Can you work these out from the drawing? Everything is in mm from the part's minimum corner. A direction names the side the tool comes from. Give positions to 0.01 mm unless a question says otherwise; leave off trailing zeros. Loops run counter-clockwise (first coordinate to the right, second up) from the corner with the lowest first, then second, coordinate; pieces in that order, holes last. Notation, with made-up numbers: (86.25, 24) - (118.25, 24) arc R21 ccw to (118.25, 63) - close; hole circle Ø6 at (-28.5, -3.75). An arc over 180 degrees is marked (long way). Answer in a Markdown table with one row per item.
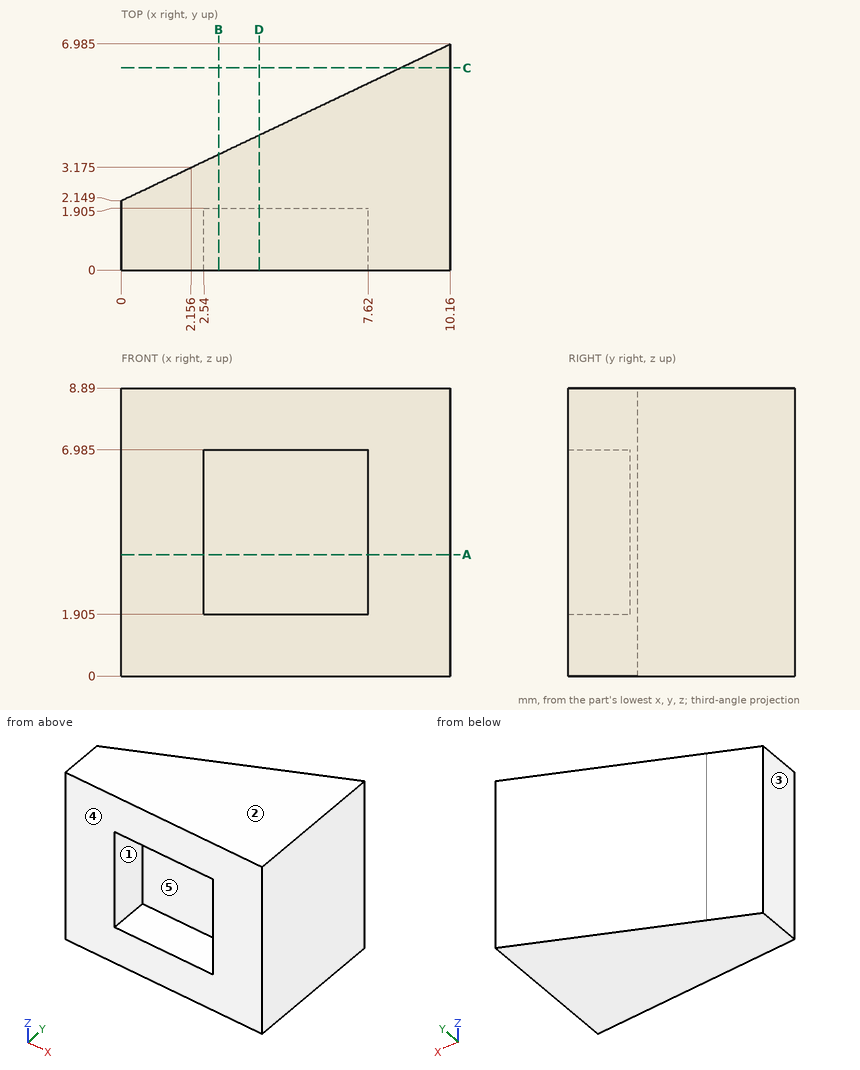
Q1. Imagine slicing it at D-D, the plane x = 4.25. Write out the boundary of the cut face in (y, z) (1 decimal), and give its area (3 significant figures).
Checked values:
| item | result |
|---|---|
| outline | (0, 0) - (4.2, 0) - (4.2, 8.9) - (0, 8.9) - (0, 7) - (1.9, 7) - (1.9, 1.9) - (0, 1.9) - close |
| area | 27.4 mm² |
Q2. If we mould it in two halves opening along Z, with no side actions, what happens to the marked faces 1, 2 and 3? For each: released by +Z, released by -Z, zero draft, split by the parting line, or undercut.
Checked values:
| item | result |
|---|---|
| face 1 | undercut |
| face 2 | released by +Z |
| face 3 | zero draft |
Q3. If I drill on line 1 (Z direction, x = 2.75, y = 1.5) (1 decimal); line 2 (Y direction, x = 3.25, z = 2.75) (1 decimal); line 3 (Y direction, x = 6, z = 6.25) (1 decimal), over which ranges is the centre line in solid material (lowest first)? Write a range as [from, to].
Checked values:
| item | result |
|---|---|
| line 1 | z = [0, 1.9], [7, 8.9] |
| line 2 | y = [1.9, 3.7] |
| line 3 | y = [1.9, 5] |
Q4. Imagine slicing it at B-B, the plane x = 3. Write out the boundary of the cut face in (y, z) (1 decimal), and give its area (3 significant figures).
Checked values:
| item | result |
|---|---|
| outline | (0, 0) - (3.6, 0) - (3.6, 8.9) - (0, 8.9) - (0, 7) - (1.9, 7) - (1.9, 1.9) - (0, 1.9) - close |
| area | 22.1 mm² |
Q5. On a 3-axis mill with a long thin cutter (end or side, diameter ignored), from which of +Z, -Z, +X, -X, +Y, -Y can I reach the whole of each face in a straight line? I mean the marked faces 4 and 5. Say none if no direction works.
Checked values:
| item | result |
|---|---|
| face 4 | +Z, -Z, +X, -X, -Y |
| face 5 | -Y |
Q6. Imagine slicing it at C-C, the plane y = 6.25. Write out the boundary of the cut face in (x, z) (1 decimal).
Checked values:
| item | result |
|---|---|
| outline | (8.6, 0) - (10.2, 0) - (10.2, 8.9) - (8.6, 8.9) - close |
Q7. For pin 1 (4 mm diameter, centred on x = 7.5, z = 4, fed in from +Y); pin 2 (1.5 mm diameter, centred on x = 5.5, z = 5, fed in from -Y) (3 decimals); pin 3 (1 mm diameter, centred on y = 3.5, z = 5.5, fed in from -X) (1 decimal), each with a flat end and sliding along its axis, tell me the tip position at first contact or that it passes through.
Checked values:
| item | result |
|---|---|
| pin 1 | stops at y = 6.67 |
| pin 2 | stops at y = 1.905 |
| pin 3 | stops at x = 1.8 |
Q8. Imagine slicing it at A-A, the plane z = 3.75. Write out the boundary of the cut face in (x, y) (1 decimal).
Checked values:
| item | result |
|---|---|
| outline | (0, 0) - (2.5, 0) - (2.5, 1.9) - (7.6, 1.9) - (7.6, 0) - (10.2, 0) - (10.2, 7) - (0, 2.1) - close |
